The model under review builds one solid part; all positions refer to its coordinate system, in mm. A direction names the side the tool comes from. Give positions to 0.01 mm unless a question says otherwise; leave off trailing zeros. Loops run counter-clockwise (first coordinate to the right, second up) from the corner with the lowest first, then second, coordinate; pieces in that order, holes last. Notation, with made-up numbers: (56.5, 66) - (95.5, 66) arc R18 ccw to (95.5, 72) - close; hole circle Ø11 at (82.5, 56.5). An arc over 180 degrees is marked (long way). Return JSON: item names as keys, results as strings. Group by question number.
from build123d import *

# Parameters (mm, degrees)
CYLINDER001_R     = 5
CYLINDER001_DEPTH = 50
CYLINDER_R        = 5
CYLINDER_DEPTH    = 50
SKETCH_W          = 280
SKETCH_H          = 180
PAD_DEPTH         = 44
SKETCH001_W       = 30
SKETCH001_H       = 54
PAD001_DEPTH      = 10
SKETCH002_W       = 400
SKETCH002_H       = 300
PAD002_DEPTH      = 10


with BuildPart() as cylinder001:
    # Cylinder001 → Cylinder001 (new body)
    with BuildSketch(Plane(origin=(-155, -66, -30), x_dir=(1, 0, 0), z_dir=(0, 0, 1))):
        Circle(CYLINDER001_R)
    extrude(amount=CYLINDER001_DEPTH)


with BuildPart() as cylinder:
    # Cylinder → Cylinder (new body)
    with BuildSketch(Plane(origin=(155, -66, -25), x_dir=(1, 0, 0), z_dir=(0, 0, 1))):
        Circle(CYLINDER_R)
    extrude(amount=CYLINDER_DEPTH)


with BuildPart() as pad:
    # Sketch → Pad (new body)
    with BuildSketch(Plane.XY):
        Rectangle(SKETCH_W, SKETCH_H)
    extrude(amount=PAD_DEPTH)


with BuildPart() as fusion:
    # Sketch001 → Pad001 (new body)
    with BuildSketch(Plane.XY):
        with Locations((155, -63)):
            Rectangle(SKETCH001_W, SKETCH001_H)
        with Locations((-155, -63)):
            Rectangle(SKETCH001_W, SKETCH001_H)
    extrude(amount=PAD001_DEPTH)

    # Fusion: union Pad
    add(pad.part)


with BuildPart() as cut001:
    # Sketch002 → Pad002 (new body)
    with BuildSketch(Plane(origin=(0, 0, -10), x_dir=(1, 0, 0), z_dir=(0, 0, -1))):
        with Locations((0, -10)):
            Rectangle(SKETCH002_W, SKETCH002_H)
    extrude(amount=-PAD002_DEPTH)

    # Fusion001: union Fusion
    add(fusion.part)

    # Cut: cut Cylinder
    add(cylinder.part, mode=Mode.SUBTRACT)

    # Cut001: cut Cylinder001
    add(cylinder001.part, mode=Mode.SUBTRACT)


solid = cut001.part
Item 1: Take a section at D-D (y = -12). State the section outline as (x, z) points, then the cut area to 3 significant figures.
Item 2: Take a section at C-C (y = -66). State the section outline as (x, z) points, then the cut area to 3 significant figures.
Item 3: For P1, Ø13, axis at x = 155, y = -66, coming from the +Z side; P2, Ø6, axis at y = 61, z = 14.5, coming from the -X side; P3, Ø1, axis at x = -137, z = 5, coming from the +Y side, all flat-tipped, find the tip position at first contact; note any pin that passes through.
Item 4: Take a section at A-A (x = -155). State the section outline as (y, z) points, then the cut area to 3 significant figures.
Item 5: Take a section at B-B (z = 5). State the section outline as (x, y) points.
Item 6: Tool access review of faces 1 (the face through (155, -57, 10)), 2 (the face through (155, -36, 5)), 3 (the face through (-170, -63, 5)): name each direction out of +Z, -Z, +X, -X, +Y, -Y from which nothing blocks a thin tool from reaching the whole face with its end or side.
Item 7: For L1, parallel to X at y = -66, z = -1; L2, parallel to X at y = -66, z = 6; L3, parallel to Y at x = -155, z = 5, list the stretches that pass through material, from the lowest coordinate up. Write a range as from..to.
Item 8: Mouldability with a two-part tool opening along Y and no side actions: class faces 4 (the face through (-159, -63, 0)), 5 (the face through (200, 12, -5)), 6 (the face through (151, -63, 0)), 7 (the face through (-3, 160, -5)) as +Y half, -Y half, draft (parallel to the pull), parting line (faces both ways), or undercut.
Check sheet entries:
{
 "1": {"outline": "(-200, -10) - (200, -10) - (200, 0) - (140, 0) - (140, 44) - (-140, 44) - (-140, 0) - (-200, 0) - close", "area": "16,300 mm^2"},
 "2": {"outline": "(-200, -10) - (-160, -10) - (-160, 10) - (-170, 10) - (-170, 0) - (-200, 0) - close; (-150, -10) - (150, -10) - (150, 10) - (140, 10) - (140, 44) - (-140, 44) - (-140, 10) - (-150, 10) - close; (160, -10) - (200, -10) - (200, 0) - (170, 0) - (170, 10) - (160, 10) - close", "area": "16,500 mm^2"},
 "3": {"P1": "stops at z = 10", "P2": "stops at x = -140", "P3": "stops at y = 90"},
 "4": {"outline": "(-140, -10) - (-71, -10) - (-71, 10) - (-90, 10) - (-90, 0) - (-140, 0) - close; (-61, -10) - (160, -10) - (160, 0) - (-36, 0) - (-36, 10) - (-61, 10) - close", "area": "3,340 mm^2"},
 "5": {"outline": "(-170, -90) - (170, -90) - (170, -36) - (140, -36) - (140, 90) - (-140, 90) - (-140, -36) - (-170, -36) - close; hole circle Ø10 at (-155, -66); hole circle Ø10 at (155, -66)"},
 "6": {"face 1": "+Z, +X, +Y, -Y", "face 2": "+Z, +X, +Y", "face 3": "+Z, -X, +Y, -Y"},
 "7": {"L1": "x = -200..-160, -150..150, 160..200", "L2": "x = -170..-160, -150..150, 160..170", "L3": "y = -90..-71, -61..-36"},
 "8": {"face 4": "undercut", "face 5": "draft", "face 6": "undercut", "face 7": "+Y half"}
}
